```python
from build123d import *

# Parameters (mm, degrees)
F1_DEPTH = 1016
F3_DEPTH = 57.151


with BuildPart() as f1:
    # F0 (on Top) → F1 (new body)
    with BuildSketch(Plane.XY):
        Polygon((57.15, 0), (0, 0), (0, -57.15), (19.05, -57.15), (19.05, -19.05), (57.15, -19.05), align=None)
    extrude(amount=F1_DEPTH)

    # F2 (on face) → F3 (cut, through all)
    with BuildSketch(Plane(origin=(0, 0, 0), x_dir=(-1, 0, 0), z_dir=(0, 1, 0))):
        Polygon((-57.15, 0), (0, 0), (-57.15, 10.077087), align=None)
        Polygon((0, 876.922422), (0, 1016), (-57.15, 1016), (-57.15, 886.999509), align=None)
    extrude(amount=-F3_DEPTH, mode=Mode.SUBTRACT)


solid = f1.part
```
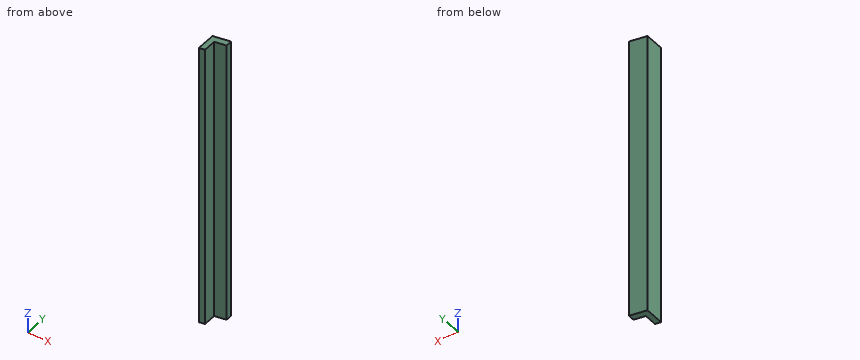
Part model, mm, in its own coordinate system. Round coordinates to 2 decimals unless told otherwise and drop trailing zeros. Order: outer loops, then holes, each group sorted by start corner. A loop starts at its lowest first (then second) coordinate and runs counter-clockwise, first axis right, second up. Notation, with made-up numbers: M -4.75,8.25 L 50.25,8.25 A13 ccw 50.25,14.25 Z; hole C 59.5,5 d11. An arc over 180 degrees is marked long. Answer in a Markdown table with one row per item. Add a question column.
Q1. Cut at B-B on y = -50. Give the cut face in (x, z).
Q2. Pin check, flat tips, straight feed: pin 1 (4 mm diameter, centred on x = 23.5, z = 317.5, fed in from -Y); pin 2 (3 mm diameter, centred on x = 50, y = -6.5, fed in from -Z); pin 3 (1.5 mm diameter, centred on y = -38, z = 435.5, fed in from +X). Stop position of each tip, or through.
Q3. Cut at C-C on x = 40. Give the cut face in (y, z).
Q4. Cut at A-A on z = 160. Give the cut face in (x, y).
Q5. Wall check: L1, parallel to Y at x = 49.5, z = 848.5; L2, parallel to X at y = -36, z = 380; L3, parallel to Z at x = 32.5, y = -3.5. Give the ranges that are in metal, low to high. Write a range as from..to.
Established:
| question | item | result |
|---|---|---|
| 1 | outline | M 0,0 L 19.05,3.36 L 19.05,880.28 L 0,876.92 Z |
| 2 | pin 1 | stops at y = -19.05 |
| 2 | pin 2 | stops at z = 8.55 |
| 2 | pin 3 | stops at x = 19.05 |
| 3 | outline | M -19.05,7.05 L 0,7.05 L 0,883.98 L -19.05,883.98 Z |
| 4 | outline | M 0,-57.15 L 19.05,-57.15 L 19.05,-19.05 L 57.15,-19.05 L 57.15,0 L 0,0 Z |
| 5 | L1 | y = -19.05..0 |
| 5 | L2 | x = 0..19.05 |
| 5 | L3 | z = 5.73..882.65 |
